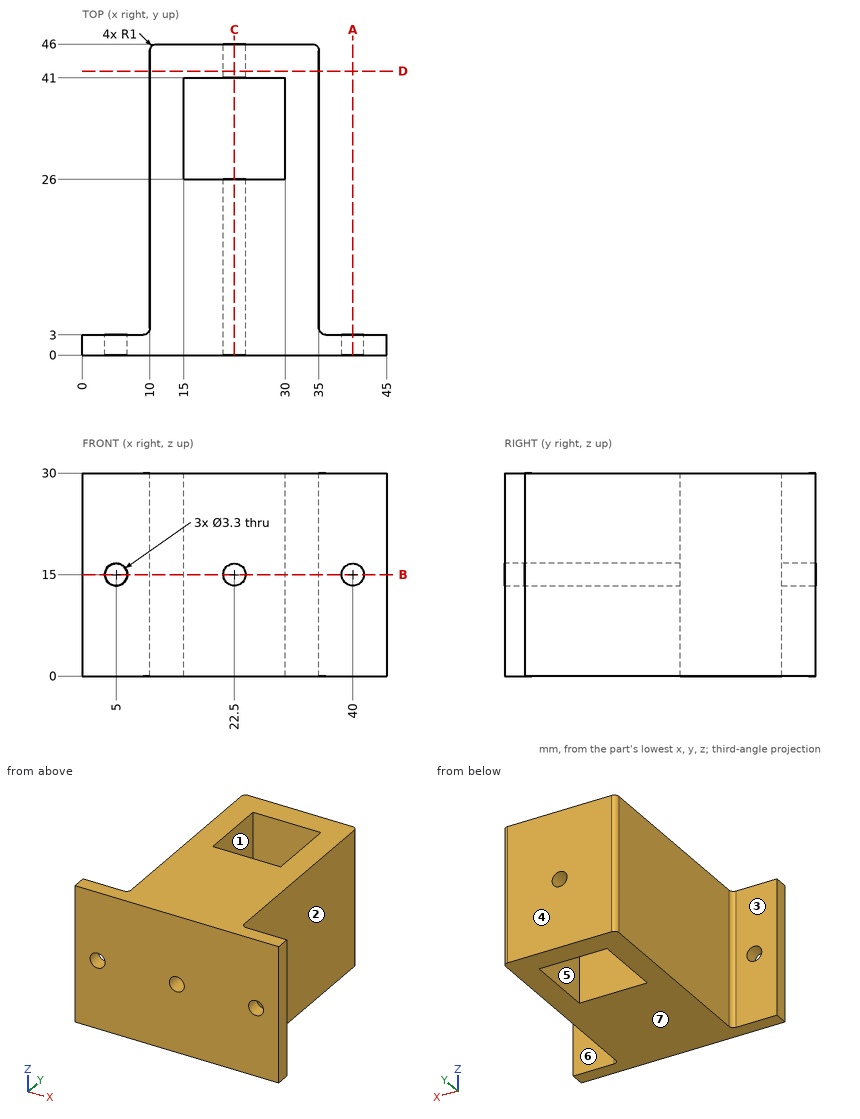
Here's the drawing with two shaded views (mm, measured from the low corner). I have some questions. A direction names the side the tool comes from. Round coordinates to 2 decimals unless told otherwise and drop trailing zeros. Loops run counter-clockwise (first coordinate to the right, second up) from the corner with the lowest first, then second, coordinate; pieces in that order, holes last. Notation, with made-up numbers: M 40,-28 L 99,-28 A28 cw 99,3 Z; hole C 12.25,28.5 d4. An arc over 180 degrees is marked long. Put each result on its own line as item: value.
Q1. For pin 1 (8 mm diameter, centred on y = 34, z = 18.5, fed in from +X); pin 2 (16.5 mm diameter, centred on y = 34.5, z = 15, fed in from -X); pin 3 (7 mm diameter, centred on x = 3, z = 13.5, fed in from +Y), each with a flat end and sliding along its axis, tell me the tip position at first contact or that it passes through.
Check result:
pin 1: x = 35
pin 2: x = 10
pin 3: y = 3
Q2. Imagine slicing it at A-A (x = 40). Write out the boundary of the cut face in (y, z).
Check result:
outline: M 0,0 L 3,0 L 3,13.35 L 0,13.35 Z; M 0,16.65 L 3,16.65 L 3,30 L 0,30 Z
Q3. I need wall thicknesses on probe 1 along X at (y, z) = (2.3, 15); probe 2 along Y at (x, z) = (29, 27.5); probe 3 along X at (y, z) = (33.5, 26.75). Which ranges of each line are inside material? Lowest first, please.
Check result:
probe 1: 0 to 3.35, 6.65 to 20.85, 24.15 to 38.35, 41.65 to 45
probe 2: 0 to 26, 41 to 46
probe 3: 10 to 15, 30 to 35
Q4. Imagine slicing it at D-D (y = 42). Write out the boundary of the cut face in (x, z).
Check result:
outline: M 10,0 L 35,0 L 35,30 L 10,30 Z; hole C 22.5,15 d3.3
Q5. Imagine slicing it at B-B (z = 15). State how many separate pieces and enclosed holes the cut face has, then the cut area to 3 significant figures.
Check result:
separate pieces: 4
enclosed holes: 0
area: 863 mm2
Q6. Imagine slicing it at C-C (x = 22.5). Write out the boundary of the cut face in (y, z).
Check result:
outline: M 0,0 L 26,0 L 26,13.35 L 0,13.35 Z; M 0,16.65 L 26,16.65 L 26,30 L 0,30 Z; M 41,0 L 46,0 L 46,13.35 L 41,13.35 Z; M 41,16.65 L 46,16.65 L 46,30 L 41,30 Z
Q7. Thinking about a two-plate mould opening in Y: for the marked faces 5, 6 and 7, which applies, released by +Y, released by -Y, zero draft, split by the parting line, or undercut?
Check result:
face 5: undercut
face 6: released by +Y
face 7: zero draft
Q8. On a 3-axis mill with a long thin cutter (end or side, diameter ignored), from which of +Z, -Z, +X, -X, +Y, -Y can I reach the whole of each face in a straight line? I mean the marked faces 1, 2, 3 and 4. Say none if no direction works.
Check result:
face 1: +Z, -Z
face 2: +Z, -Z, +X, +Y
face 3: +Z, -Z, -X, +Y
face 4: +Z, -Z, +X, -X, +Y
